```python
from build123d import *

# Parameters (mm, degrees)
F0_W      = 12
F0_H      = 12
F1_DEPTH  = 20
F2_R      = 5
F3_DEPTH  = 5
F4_R      = 9
F5_DEPTH  = 30
F8_DEPTH  = 2
F10_D     = 8
F10_DEPTH = 20
F10_TIP   = 2.4034424761
F11_SIZE  = 1.5


with BuildPart() as f1:
    # F0 (on Top) → F1 (new body, symmetric)
    with BuildSketch(Plane.XY):
        Rectangle(F0_W, F0_H)
    extrude(amount=F1_DEPTH, both=True)

    # F2 (on face) → F3 (join)
    with BuildSketch(Plane.XY.offset(20)):
        Circle(F2_R)
    extrude(amount=F3_DEPTH)

    # F4 (on face) → F5 (join)
    with BuildSketch(Plane(origin=(0, 0, -20), x_dir=(1, 0, 0), z_dir=(0, 0, -1))):
        Circle(F4_R)
    extrude(amount=F5_DEPTH)

    # F7 (on offset) → F8 (cut)
    with BuildSketch(Plane.YZ.offset(9)):
        with BuildLine():
            Line((-3, -36), (-3, -42))
            ThreePointArc((-3, -42), (0, -45), (3, -42))
            Line((3, -42), (3, -36))
            ThreePointArc((3, -36), (0, -33), (-3, -36))
        make_face()
    extrude(amount=-F8_DEPTH, mode=Mode.SUBTRACT)

    # F10
    with Locations(Plane(origin=(0, 0, -50), x_dir=(1, 0, 0), z_dir=(0, 0, -1))):
        with Locations((0, 0)):
            Hole(F10_D / 2, depth=F10_DEPTH)
            with Locations((0, 0, -(F10_DEPTH + F10_TIP / 2))):  # 118° drill point
                Cone(0, F10_D / 2, F10_TIP, mode=Mode.SUBTRACT)

    # F11
    f11_edges = [f1.edges().sort_by_distance(p)[0] for p in [
        (-9, 0, -50),
    ]]
    chamfer(f11_edges, length=F11_SIZE)


solid = f1.part
```
Build history of the part. All positions in model axes, mm. A direction names the side the tool comes from. Give positions to 0.01 mm unless a question says otherwise; leave off trailing zeros. Loops run counter-clockwise (first coordinate to the right, second up) from the corner with the lowest first, then second, coordinate; pieces in that order, holes last.
1) Band-saw the part on B-B on z = 14. List the corners of the cut face in (x, y), then the cut area to 3 significant figures.
Values follow:
outline: (-6, -6) - (6, -6) - (6, 6) - (-6, 6) - close
area: 144 mm2
2) 3-axis set-ups, long thin cutter, end or side, ignore diameter. For faces 1 (the face through (-6, 0, 0)), 2 (the face through (8, 0, -45)), 3 (the face through (0.867, 3.905, -39.86)), 4 (the face through (6, 0, 0)), 5 (the face through (5.2, 0.1, 20)): which of +Z, -Z, +X, -X, +Y, -Y reach the whole face in a straight line?
Values follow:
face 1: +Z, -X, +Y, -Y
face 2: +X
face 3: -Z
face 4: +Z, +X, +Y, -Y
face 5: +Z
3) Probe line 1 along Y through (x, z) = (0, -36.5); line 2 along Z through (x, y) = (1.25, -6.5); line 3 along Z through (x, y) = (5.5, 2.75). List the from-to ranges inside material, lowest first.
Values follow:
line 1: y = -9 to -4, 4 to 9
line 2: z = -50 to -20
line 3: z = -50 to 20
4) Two-plate mould, pull along Y, no slides. Class faces 6 (the face through (0, 6, 0)), 7 (the face through (-0.151, 0.678, -28.014)), 8 (the face through (8, 0, -33)), 9 (the face through (0, -6, 0)): released by +Y, released by -Y, zero draft, split by the parting line, or undercut.
Values follow:
face 6: released by +Y
face 7: undercut
face 8: undercut
face 9: released by -Y
5) Drop flat-ended pins along their axis: P1, Ø3.5, axis at x = -0.5, z = -9, coming from the +Y side; P2, Ø2, axis at y = 1.5, z = -34, coming from the +X side; P3, Ø1.2, axis at x = 7.5, z = -40, coming from the +Y side. Give the stop position or say it passes through.
Values follow:
P1: stops at y = 6
P2: stops at x = 8.95
P3: stops at y = 5.78
6) Band-saw the part on A-A on z = -41. List the corners of the cut face in (x, y).
Values follow:
outline: (7, -3) - (7, 3) - (8.49, 3) arc R9 ccw (long way) to (8.49, -3) - close; hole circle Ø8 at (0, 0)
